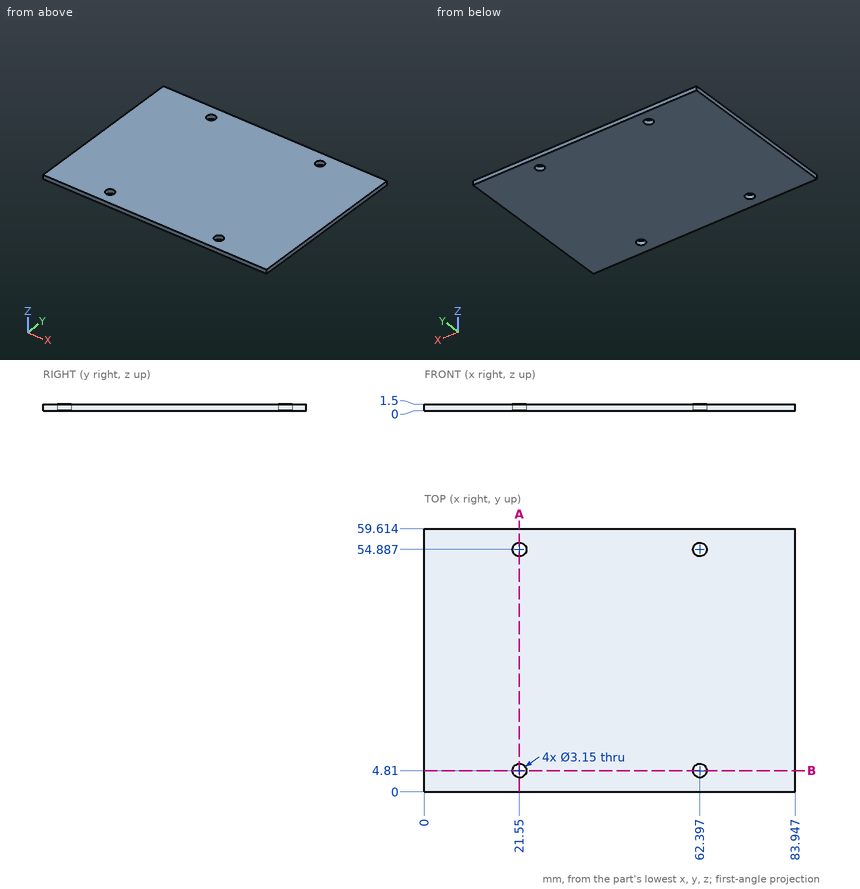
Design review of the part shown in the three views and the two pictorial views. Dimensions are in mm from the part's minimum x, y and z. Give positions to 0.01 mm unless a question says otherwise; leave off trailing zeros. Write each loop counter-clockwise with the first axis right and the second up, starting at its lowest first coordinate (ties: lowest second). Pieces come first, ordered by that corner, then holes.
Item 1: Take a section at B-B (y = 4.81). Give the boundary of the cut face in (x, z) (3 decimals).
Item 2: Take a section at A-A (x = 21.55). Give the boundary of the cut face in (y, z) (1 decimal).
Item 3: Insertion check: P1, Ø2.5, axis at x = 21.55, y = 54.89, coming from the +Z side. The pin has a flat end and moves straight along its axis. Give the tip position at first contact, or say it passes through.
Item 4: Wall thickness on probe 1 along X at (y, z) = (5, 0.9); probe 2 along Y at (x, z) = (21.55, 0.55) (1 decimal); probe 3 along X at (y, z) = (55.5, 0.85): over which ranges is each line inside the solid? List them lowest first.
Established:
1. outline: (0, 0) - (19.975, 0) - (19.975, 1.5) - (0, 1.5) - close; (23.125, 0) - (60.822, 0) - (60.822, 1.5) - (23.125, 1.5) - close; (63.972, 0) - (83.947, 0) - (83.947, 1.5) - (63.972, 1.5) - close
2. outline: (0, 0) - (3.2, 0) - (3.2, 1.5) - (0, 1.5) - close; (6.4, 0) - (53.3, 0) - (53.3, 1.5) - (6.4, 1.5) - close; (56.5, 0) - (59.6, 0) - (59.6, 1.5) - (56.5, 1.5) - close
3. P1: passes through
4. probe 1: x = 0 to 19.99, 23.11 to 60.83, 63.96 to 83.95
4. probe 2: y = 0 to 3.2, 6.4 to 53.3, 56.5 to 59.6
4. probe 3: x = 0 to 20.1, 23 to 60.95, 63.85 to 83.95
